```python
from build123d import *

# Parameters (mm, degrees)
F0_W     = 98.7017413428
F0_H     = 98.2726
F0_R     = 40.4346760416
F1_DEPTH = 50.8
F2_R     = 48.8166771829
F2_R_2   = 40.4346760416
F3_DEPTH = 148.2671336


# Not quite as in the source:
# - an extrude ends at something that could not be found from the text; its depth is read off the source's solid


with BuildPart() as f1:
    # F0 (on Front) → F1 (new body)
    with BuildSketch(Plane.XZ):
        Rectangle(F0_W, F0_H)
        Circle(F0_R, mode=Mode.SUBTRACT)
    extrude(amount=-F1_DEPTH)

    # F2 (on face) → F3 (join, through all)
    with BuildSketch(Plane.XZ):
        Circle(F2_R)
        Circle(F2_R_2, mode=Mode.SUBTRACT)
    extrude(amount=F3_DEPTH)


solid = f1.part
```
For this review, take the finished solid that the model builds, in its own axes (mm). A direction names the side the tool comes from. Coordinates: 2 decimals unless noted, no trailing zeros. Order: outer loops, then holes, each group sorted by start corner. A loop starts at its lowest first (then second) coordinate and runs counter-clockwise, first axis right, second up. Notation, with made-up numbers: (56, -34.5) - (109, -34.5) arc R11 ccw to (109, -30.5) - close; hole circle Ø4 at (70, 80.25). An arc over 180 degrees is marked (long way). Answer as a JSON object with one key per item and string values. Group by question number.
1. We need section D-D on y = -83. State the section outline as (x, z) points.
2. Clearance check with flat-ended pins moving along their axes: P1, Ø6, axis at y = -41, z = -1.5, coming from the +X side; P2, Ø1.5, axis at y = -104.5, z = -28, coming from the -X side; P3, Ø5, axis at x = 30.5, y = -13, coming from the -Z side. State where each tip first meets the part, or that it passes through.
3. We need section B-B on z = 0. State the section outline as (x, y) points.
4. For faces 5 (the flat face through (-34, 50.8, 23)), 6 (the cylindrical face through (-48.77, -73.1, 2.15)), list the 3-axis set-ups (+Z, -Z, +X, -X, +Y, -Y) from which the entire face can be reached by the end or side of a thin tool; tool diameter is ignored.
5. We need section C-C on z = 43. State the section outline as (x, y) points, then the cut area to 3 significant figures.
6. For probe 1 along Z at (x, y) = (0, -56.5); probe 2 along Z at (x, y) = (19.5, 19); probe 3 along X at (y, z) = (-101, 9.5), list the stretches that pass through material, from the lowest coordinate up.
7. We need section A-A on x = 0. State the section outline as (y, z) points, then the cut area to 3 significant figures.
8. The part is to be moulded in two halves that separate along Z. For faces 1 (the flat face through (-1, 25, -49.136)), 2 (the flat face through (49.351, 25, -1)), 3 (the cylindrical face through (-8.765, -47.34, -39.473)), 4 (the flat face through (-1, 25, 49.136)), say which applies: pulls with the +Z half, pulls with the -Z half, needs draft (parallel to the pull), parting line crosses it, or undercut.
Final values:
{
 "1": {"outline": "circle Ø97.63 at (0, 0); hole circle Ø80.87 at (0, 0)"},
 "2": {"P1": "x = 48.82", "P2": "x = -40.5", "P3": "z = -39.99"},
 "3": {"outline": "(-49.35, 0) - (-48.82, 0) - (-48.82, -148.27) - (-40.43, -148.27) - (-40.43, 50.8) - (-49.35, 50.8) - close; (40.43, -148.27) - (48.82, -148.27) - (48.82, 0) - (49.35, 0) - (49.35, 50.8) - (40.43, 50.8) - close"},
 "4": {"face 5": "+Z, -Z, +X, -X, +Y", "face 6": "-Y"},
 "5": {"outline": "(-49.35, 0) - (-23.11, 0) - (-23.11, -148.27) - (23.11, -148.27) - (23.11, 0) - (49.35, 0) - (49.35, 50.8) - (-49.35, 50.8) - close", "area": "11,900 mm²"},
 "6": {"probe 1": "-48.82 to -40.43, 40.43 to 48.82", "probe 2": "-49.14 to -35.42, 35.42 to 49.14", "probe 3": "-47.88 to -39.3, 39.3 to 47.88"},
 "7": {"outline": "(-148.27, -48.82) - (0, -48.82) - (0, -49.14) - (50.8, -49.14) - (50.8, -40.43) - (-148.27, -40.43) - close; (-148.27, 40.43) - (50.8, 40.43) - (50.8, 49.14) - (0, 49.14) - (0, 48.82) - (-148.27, 48.82) - close", "area": "3,370 mm²"},
 "8": {"face 1": "pulls with the -Z half", "face 2": "needs draft", "face 3": "undercut", "face 4": "pulls with the +Z half"}
}
